The listing builds one solid part. Answer for the finished solid, in the listing's coordinates (mm). A direction names the side the tool comes from. Coordinates: 2 decimals unless noted, no trailing zeros. Order: outer loops, then holes, each group sorted by start corner. A loop starts at its lowest first (then second) coordinate and runs counter-clockwise, first axis right, second up. Notation, with made-up numbers: (12, -33.75) -> (67, -33.75) arc R27 ccw to (67, 2.25) -> close; hole circle Ø10 at (-2.5, 44). An arc over 180 degrees is marked (long way). Return JSON: item names as keys, results as strings.
Autodesk Inventor part; units mm, degrees
ref_plane "YZ Plane" through (0, 0, 0) normal (1, 0, 0) x (0, 1, 0)
ref_plane "XZ Plane" through (0, 0, 0) normal (0, 1, 0) x (-1, 0, 0)
ref_plane "XY Plane" through (0, 0, 0) normal (0, 0, 1) x (1, 0, 0)
sketch "Sketch1" plane through (0, 0, 0) normal (0, 0, 1) x (1, 0, 0)
  circle A0 centre (0, 0) radius 3.175
  line L0 (-2.2451, 2.2451) -> (2.2451, 2.2451)
  line L1 (2.2451, 2.2451) -> (2.2451, -2.2451)
  line L2 (2.2451, -2.2451) -> (-2.2451, -2.2451)
  line L3 (-2.2451, -2.2451) -> (-2.2451, 2.2451)
  line L4 (-2.2451, 2.2451) -> (2.2451, -2.2451) construction
  line L5 (2.2451, 2.2451) -> (-2.2451, -2.2451) construction
  dimension "d0" = 6.35
  dimension "d6" = 4.4901
  dimension "d7" = 4.4901
extrude "Extrusion1" add sketch "Sketch1" along normal blind 139.7
extrude "Extrusion2" cut sketch "Sketch1" along normal blind 3.175 contours A0 L1 | L0 A0 | A0 L2 | L3 A0
ref_plane "Work Plane1" through (0, 0, 139.7) normal (0, 0, -1) x (-1, 0, 0)
sketch "Sketch2" plane through (0, 0, 139.7) normal (0, 0, -1) x (-1, 0, 0)
  line L0 (-2.2451, 2.2451) -> (-2.2451, -2.2451)
  line L1 (2.2451, 2.2451) -> (-2.2451, 2.2451)
  line L2 (-2.2451, 2.2451) -> (-2.2451, -2.2451)
  line L3 (-2.2451, -2.2451) -> (2.2451, -2.2451)
  line L4 (2.2451, -2.2451) -> (2.2451, 2.2451)
  line L5 (2.2451, 2.2451) -> (-2.2451, -2.2451) construction
  line L6 (-2.2451, 2.2451) -> (2.2451, -2.2451) construction
  circle A0 centre (0, 0) radius 3.175
  dimension "d11" = 4.4901
  dimension "d12" = 4.4901
  dimension "d13" = 6.35
extrude "Extrusion3" cut sketch "Sketch2" along normal blind 3.175 contours A0 L1 | L0 A0 | L3 A0 | A0 L4
ref_plane "Work Plane2" through (0, 0, 46.99) normal (0, 0, 1) x (1, 0, 0)
sketch "Sketch3" plane through (0, 0, 46.99) normal (0, 0, 1) x (1, 0, 0)
  circle A0 centre (0, 0) radius 3.175
  line L0 (-2.2451, 2.2451) -> (2.2451, 2.2451)
  line L1 (2.2451, 2.2451) -> (2.2451, -2.2451)
  line L2 (2.2451, -2.2451) -> (-2.2451, -2.2451)
  line L3 (-2.2451, -2.2451) -> (-2.2451, 2.2451)
  line L4 (-2.2451, 2.2451) -> (2.2451, -2.2451) construction
  line L5 (2.2451, 2.2451) -> (-2.2451, -2.2451) construction
  dimension "d17" = 4.4901
  dimension "d18" = 4.4901
extrude "Extrusion4" cut sketch "Sketch3" against normal blind 3.302 contours A0 L1 | L0 A0 | A0 L2 | L3 A0
properties part number "rod"
Item 1: The part is cut by section A-A on y = 0. Determine the outline of the cut face in (x, z) (3 decimals).
Answer list:
{"outline": "(-3.175, 3.175) -> (-2.245, 3.175) -> (-2.245, 0) -> (2.245, 0) -> (2.245, 3.175) -> (3.175, 3.175) -> (3.175, 43.688) -> (2.245, 43.688) -> (2.245, 46.99) -> (3.175, 46.99) -> (3.175, 136.525) -> (2.245, 136.525) -> (2.245, 139.7) -> (-2.245, 139.7) -> (-2.245, 136.525) -> (-3.175, 136.525) -> (-3.175, 46.99) -> (-2.245, 46.99) -> (-2.245, 43.688) -> (-3.175, 43.688) -> close"}
Item 2: Flat-ended cylindrical pins translate along their axes: pin 1 (1 mm diameter, centred on y = 0, z = 45.5, fed in from +X); pin 2 (0.7 mm diameter, centred on x = 3, y = 0.5, fed in from +Z) (3 decimals); pin 3 (3.5 mm diameter, centred on x = 0.5, z = 1, fed in from +Y). Find the tip coordinate at first contact, or state that the pin passes through.
Answer list:
{"pin 1": "x = 2.25", "pin 2": "z = 136.525", "pin 3": "y = 2.25"}
Item 3: The part is cut by section C-C on z = 81. Determine the outline of the cut face in (x, y) (3 decimals), plus the area to 3 significant figures.
Answer list:
{"outline": "circle Ø6.35 at (0, 0)", "area": "31.7 mm2"}
Item 4: Find the intervals of material crossed by probe 1 along Z at (x, y) = (-0.5, -2.5) (3 decimals); probe 2 along Y at (x, z) = (0.25, 63), in increasing order.
Answer list:
{"probe 1": "3.175 to 43.688, 46.99 to 136.525", "probe 2": "-3.17 to 3.17"}
Item 5: Determine the mould class of faces 1 (the flat face through (0, 2.245, 45)), 2 (the flat face through (0, 0, 139.7)), 3 (the flat face through (-2.245, 0, 45)), 4 (the flat face through (2.245, 0, 138)) for opening direction Z: pulls with the +Z half, pulls with the -Z half, needs draft (parallel to the pull), parting line crosses it, or undercut.
Answer list:
{"face 1": "undercut", "face 2": "pulls with the +Z half", "face 3": "undercut", "face 4": "needs draft"}
Item 6: Which of the six approach directions +Z, -Z, +X, -X, +Y, -Y give full straight-line access (tool end or side, diameter ignored) to faces 5 (the flat face through (0, -2.245, 2)), 6 (the flat face through (0, -2.245, 138)), 7 (the flat face through (0, 2.245, 138))?
Answer list:
{"face 5": "-Z, +X, -X, -Y", "face 6": "+Z, +X, -X, -Y", "face 7": "+Z, +X, -X, +Y"}
